Design review of the part built by this model. Coordinates are the model's own, in mm. Coordinates: 2 decimals unless noted, no trailing zeros. Write each loop counter-clockwise with the first axis right and the second up, starting at its lowest first coordinate (ties: lowest second). Pieces come first, ordered by that corner, then holes.
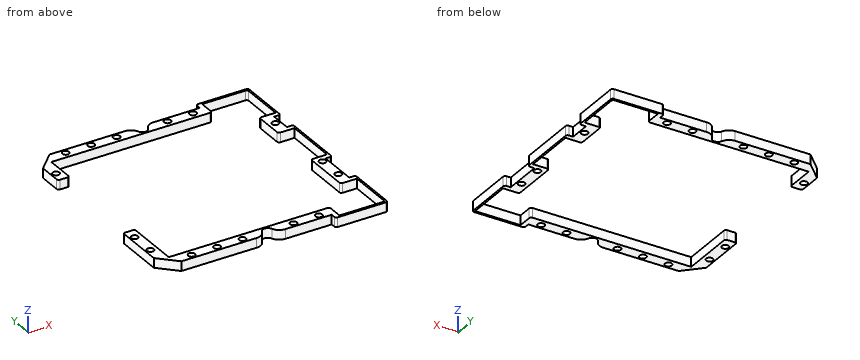
```python
from build123d import *

# Parameters (mm, degrees)
SKETCH1_R           = 3.38
BOSS_EXTRUDE1_DEPTH = 9.525
FILLET1_R           = 10
FILLET2_R           = 2


with BuildPart() as part:
    # Sketch1 → Boss-Extrude1 (new body)
    # profile 1 of 7: a face of its own
    with BuildSketch(Plane.XY):
        Polygon((212.852, -66.426), (212.852, -71.426), (217.352, -71.426), (217.352, -123.926), (212.852, -123.926), (212.852, -128.926), (219.202, -128.926), (219.202, -66.426), align=None)
    # profile 2 of 7: a face of its own
    with BuildSketch(Plane.XY):
        Polygon((212.852, -40.7759), (201.238585453, -40.7759), (201.238585453, -71.426), (212.852, -71.426), (212.852, -66.426), (212.852, -45.7759), align=None)
        with Locations(Location((208.026, -55.626, 0), (0, 0, 180))):
            Circle(SKETCH1_R, mode=Mode.SUBTRACT)
    # profile 3 of 7: a face of its own
    with BuildSketch(Plane.XY):
        Polygon((212.852, -123.926), (201.238585453, -123.926), (201.238585453, -172.0761), (212.852, -172.0761), (212.852, -167.0761), (212.852, -128.926), align=None)
        with Locations(Location((208.026, -157.226, 0), (0, 0, 180))):
            Circle(SKETCH1_R, mode=Mode.SUBTRACT)
        with Locations(Location((208.026, -131.826, 0), (0, 0, 180))):
            Circle(SKETCH1_R, mode=Mode.SUBTRACT)
    # profile 4 of 7: a face of its own
    with BuildSketch(Plane.XY):
        Polygon((172.0761, -217.352), (172.0761, -212.852), (167.0761, -212.852), (167.0761, -219.202), (219.202, -219.202), (219.202, -167.0761), (212.852, -167.0761), (212.852, -172.0761), (217.352, -172.0761), (217.352, -217.352), align=None)
    # profile 5 of 7: a face of its own
    with BuildSketch(Plane.XY):
        Polygon((167.0761, 0), (172.0761, 0), (172.0761, 4.5), (217.352, 4.5), (217.352, -40.7759), (212.852, -40.7759), (212.852, -45.7759), (219.202, -45.7759), (219.202, 6.35), (167.0761, 6.35), align=None)
    # profile 6 of 7: a face of its own
    with BuildSketch(Plane.XY):
        with BuildLine():
            Line((11.613414547, -41.101), (11.613414547, -11.613414547))
            Line((11.613414547, -11.613414547), (172.0761, -11.613414547))
            Line((172.0761, -11.613414547), (172.0761, 0))
            Line((172.0761, 0), (167.0761, 0))
            Line((167.0761, 0), (108.347061293, 0))
            ThreePointArc((108.347061293, 0), (110.724797574, -1.910336798), (111.6203, -4.826))
            ThreePointArc((111.6203, -4.826), (103.510336798, -9.124797574), (104.504938707, 0))
            Line((104.504938707, 0), (16.997849507, 0))
            Line((16.997849507, 0), (0, -16.997849507))
            Line((0, -16.997849507), (0, -41.101))
            Line((0, -41.101), (11.613414547, -41.101))
        make_face()
        with Locations(Location((4.826, -30.226, 0), (0, 0, 180))):
            Circle(SKETCH1_R, mode=Mode.SUBTRACT)
        with Locations(Location((30.226, -4.826, 0), (0, 0, 180))):
            Circle(SKETCH1_R, mode=Mode.SUBTRACT)
        with Locations(Location((55.626, -4.826, 0), (0, 0, 180))):
            Circle(SKETCH1_R, mode=Mode.SUBTRACT)
        with Locations(Location((81.026, -4.826, 0), (0, 0, 180))):
            Circle(SKETCH1_R, mode=Mode.SUBTRACT)
        with Locations(Location((131.826, -4.826, 0), (0, 0, 180))):
            Circle(SKETCH1_R, mode=Mode.SUBTRACT)
        with Locations(Location((157.226, -4.826, 0), (0, 0, 180))):
            Circle(SKETCH1_R, mode=Mode.SUBTRACT)
    # profile 7 of 7: a face of its own
    with BuildSketch(Plane.XY):
        with BuildLine():
            Line((11.613414547, -201.238585453), (11.613414547, -146.351))
            Line((11.613414547, -146.351), (0, -146.351))
            Line((0, -146.351), (0, -195.854150493))
            Line((0, -195.854150493), (16.997849507, -212.852))
            Line((16.997849507, -212.852), (104.504938707, -212.852))
            ThreePointArc((104.504938707, -212.852), (103.510336798, -203.727202426), (111.6203, -208.026))
            ThreePointArc((111.6203, -208.026), (110.724797574, -210.941663202), (108.347061293, -212.852))
            Line((108.347061293, -212.852), (167.0761, -212.852))
            Line((167.0761, -212.852), (172.0761, -212.852))
            Line((172.0761, -212.852), (172.0761, -201.238585453))
            Line((172.0761, -201.238585453), (11.613414547, -201.238585453))
        make_face()
        with Locations(Location((30.226, -208.026, 0), (0, 0, 180))):
            Circle(SKETCH1_R, mode=Mode.SUBTRACT)
        with Locations(Location((4.826, -182.626, 0), (0, 0, 180))):
            Circle(SKETCH1_R, mode=Mode.SUBTRACT)
        with Locations(Location((55.626, -208.026, 0), (0, 0, 180))):
            Circle(SKETCH1_R, mode=Mode.SUBTRACT)
        with Locations(Location((81.026, -208.026, 0), (0, 0, 180))):
            Circle(SKETCH1_R, mode=Mode.SUBTRACT)
        with Locations(Location((4.826, -157.226, 0), (0, 0, 180))):
            Circle(SKETCH1_R, mode=Mode.SUBTRACT)
        with Locations(Location((131.826, -208.026, 0), (0, 0, 180))):
            Circle(SKETCH1_R, mode=Mode.SUBTRACT)
        with Locations(Location((157.226, -208.026, 0), (0, 0, 180))):
            Circle(SKETCH1_R, mode=Mode.SUBTRACT)
    extrude(amount=BOSS_EXTRUDE1_DEPTH)

    # Fillet1
    fillet1_edges = [part.edges().sort_by_distance(p)[0] for p in [
        (108.347061293, -212.852, 4.7625),
        (104.504938707, -212.852, 4.7625),
        (104.504938707, 0, 4.7625),
        (108.347061293, 0, 4.7625),
    ]]
    fillet(fillet1_edges, radius=FILLET1_R)

    # Fillet2
    fillet2_edges = [part.edges().sort_by_distance(p)[0] for p in [
        (219.202, -128.926, 4.7625),
        (219.202, -167.0761, 4.7625),
        (219.202, -219.202, 4.7625),
        (167.0761, -219.202, 4.7625),
        (0, -146.351, 4.7625),
        (11.613414547, -146.351, 4.7625),
        (172.0761, -201.238585453, 4.7625),
        (201.238585453, -172.0761, 4.7625),
        (201.238585453, -123.926, 4.7625),
        (201.238585453, -71.426, 4.7625),
        (201.238585453, -40.7759, 4.7625),
        (217.352, 4.5, 4.7625),
        (172.0761, -11.613414547, 4.7625),
        (11.613414547, -41.101, 4.7625),
        (0, -41.101, 4.7625),
        (167.0761, 6.35, 4.7625),
        (219.202, 6.35, 4.7625),
        (219.202, -45.7759, 4.7625),
        (219.202, -66.426, 4.7625),
    ]]
    fillet(fillet2_edges, radius=FILLET2_R)


solid = part.part
```
(1) Consider section C-C (y = -118.5). Give the boundary of the cut face in (x, z) (3 decimals), plus the area to 3 significant figures.
(2) Consider section D-D (z = 6.25). State how many separate pieces and enclosed holes the cut face has, plus the area to 3 significant figures.
(3) Consider section B-B (x = 30). Give the boundary of the cut face in (y, z) (3 decimals).
(4) Wall thickness on line 1 (X direction, y = -36.5, z = 8.25); line 2 (Y direction, x = 124, z = 3); line 3 (Y direction, x = 30, z = 5.5): over which ranges is each line inside the solid? List them lowest first.
(5) Consider section A-A (x = 142). Give the boundary of the cut face in (y, z) (3 decimals).
(6) Insertion check: pin 1 Ø3 at (x, z) = (49, 7) entering from +Y; pin 2 Ø1 at (x, z) = (97, 8) entering from -Y; pin 3 Ø1.5 at (y, z) = (-70.5, 4) entering from -X (3 decimals). Each pin has a flat end and moves straight along its axis. Give the tip position at first contact, or say it passes through.
Results:
1. outline: (217.352, 0) - (219.202, 0) - (219.202, 9.525) - (217.352, 9.525) - close
1. area: 17.6 mm2
2. separate pieces: 1
2. enclosed holes: 16
2. area: 5,400 mm2
3. outline: (-212.852, 0) - (-211.398, 0) - (-211.398, 9.525) - (-212.852, 9.525) - close; (-204.654, 0) - (-201.239, 0) - (-201.239, 9.525) - (-204.654, 9.525) - close; (-11.613, 0) - (-8.198, 0) - (-8.198, 9.525) - (-11.613, 9.525) - close; (-1.454, 0) - (0, 0) - (0, 9.525) - (-1.454, 9.525) - close
4. line 1: x = 0 to 11.61, 217.35 to 219.2
4. line 2: y = -212.85 to -201.24, -11.61 to 0
4. line 3: y = -212.85 to -211.4, -204.65 to -201.24, -11.61 to -8.2, -1.45 to 0
5. outline: (-212.852, 0) - (-201.239, 0) - (-201.239, 9.525) - (-212.852, 9.525) - close; (-11.613, 0) - (0, 0) - (0, 9.525) - (-11.613, 9.525) - close
6. pin 1: stops at y = 0
6. pin 2: stops at y = -211.85
6. pin 3: stops at x = 201.265
